Here's the drawing with two shaded views (mm, measured from the low corner). I have some questions. A direction names the side the tool comes from. Give positions to 0.01 mm unless a question says otherwise; leave off trailing zeros. Write each loop counter-clockwise with the first axis right and the second up, starting at its lowest first coordinate (ties: lowest second). Pieces come first, ordered by that corner, then holes. Notation, with made-up numbers: (12.25, 31) - (44.25, 31) arc R15 cw to (44.25, 41) - close; hole circle Ø7 at (-32, 70.25). An arc over 180 degrees is marked (long way). Use one line per item in the form item = value.
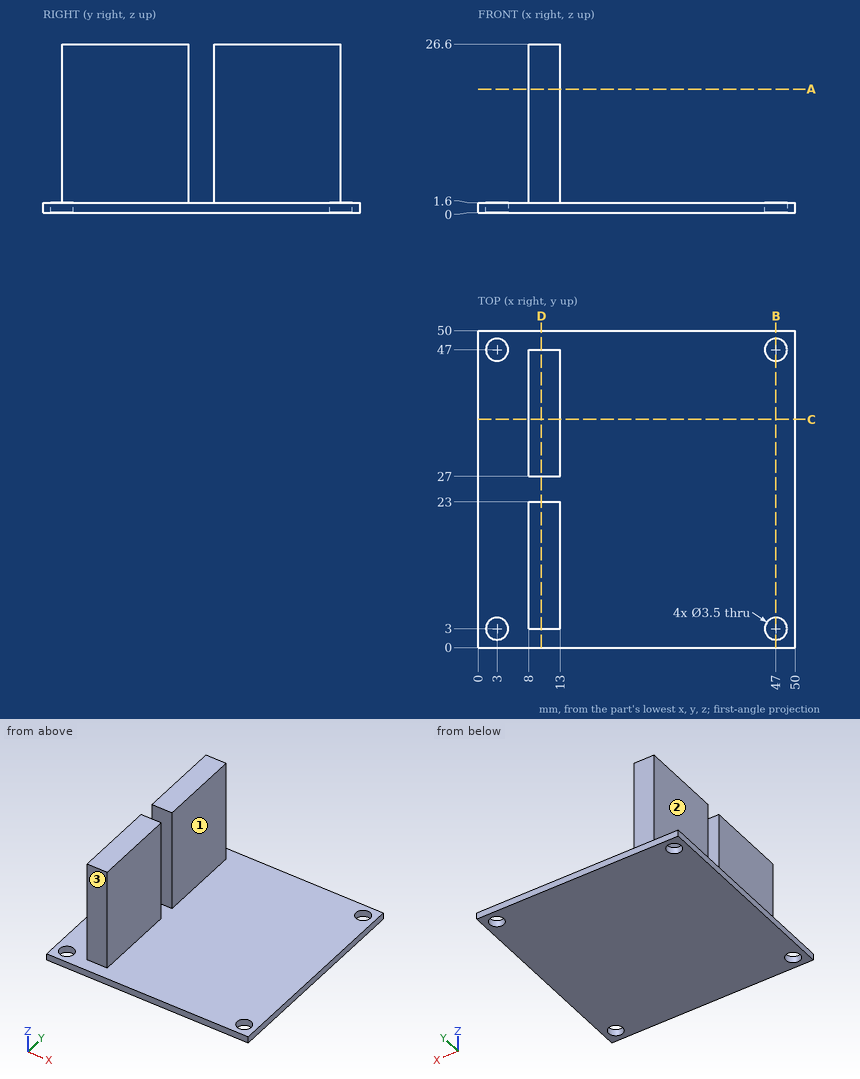
1. For pin 1 (12 mm diameter, centred on y = 39, z = 23, fed in from -X); pin 2 (15 mm diameter, centred on x = 23, y = 23.5, fed in from +Z); pin 3 (3 mm diameter, centred on x = 3, y = 47, fed in from +Z); pin 4 (4 mm diameter, centred on x = 10, z = 12.5, fed in from +Y), each with a flat end and sliding along its axis, tell me the tip position at first contact or that it passes through.
Response values:
pin_1 = 8
pin_2 = 1.6
pin_3 = through
pin_4 = 47
2. Which directions (+Z, -Z, +X, -X, +Y, -Y) give clear straight access to the entire face, cutting with the end or side of a thin tool? Please do the marked faces 1, 2 and 3.
Response values:
face_1 = +Z, +X, +Y, -Y
face_2 = +Z, -X, +Y, -Y
face_3 = +Z, +X, -X, -Y
3. Imagine slicing it at C-C, the plane y = 36. List the corners of the cut face in (x, z) for me, and give its area (3 significant figures).
Response values:
outline = (0, 0) - (50, 0) - (50, 1.6) - (13, 1.6) - (13, 26.6) - (8, 26.6) - (8, 1.6) - (0, 1.6) - close
area = 205 mm²
4. Imagine slicing it at D-D, the plane x = 10. List the corners of the cut face in (y, z) for me.
Response values:
outline = (0, 0) - (50, 0) - (50, 1.6) - (47, 1.6) - (47, 26.6) - (27, 26.6) - (27, 1.6) - (23, 1.6) - (23, 26.6) - (3, 26.6) - (3, 1.6) - (0, 1.6) - close
5. Imagine slicing it at A-A, the plane z = 19.5. List the corners of the cut face in (x, y) for me, and give its area (3 significant figures).
Response values:
outline = (8, 3) - (13, 3) - (13, 23) - (8, 23) - close; (8, 27) - (13, 27) - (13, 47) - (8, 47) - close
area = 200 mm²
6. If I drill on line 1 (Y direction, x = 3, z = 0.85); line 2 (Y direction, x = 8.5, z = 22); line 3 (Z direction, x = 45, y = 46), over which ranges is the centre line in solid material (lowest first)? Write a range as from..to.
Response values:
line_1 = 0..1.25, 4.75..45.25, 48.75..50
line_2 = 3..23, 27..47
line_3 = 0..1.6
7. Imagine slicing it at B-B, the plane x = 47. List the corners of the cut face in (y, z) for me.
Response values:
outline = (0, 0) - (1.25, 0) - (1.25, 1.6) - (0, 1.6) - close; (4.75, 0) - (45.25, 0) - (45.25, 1.6) - (4.75, 1.6) - close; (48.75, 0) - (50, 0) - (50, 1.6) - (48.75, 1.6) - close
